Geometry check sheet. Reference: drawing and pictorial views, mm from the part's lowest x, y, z. A direction names the side the tool comes from. Give positions to 0.01 mm unless a question says otherwise; leave off trailing zeros. Loops run counter-clockwise (first coordinate to the right, second up) from the corner with the lowest first, then second, coordinate; pieces in that order, holes last. Notation, with made-up numbers: (30.5, 41.25) - (69.5, 41.25) arc R7 ccw to (69.5, 49.25) - close; hole circle Ø7 at (-36.75, -9). An arc over 180 degrees is marked (long way). Use CSV: the item, a comma, the result in double quotes.
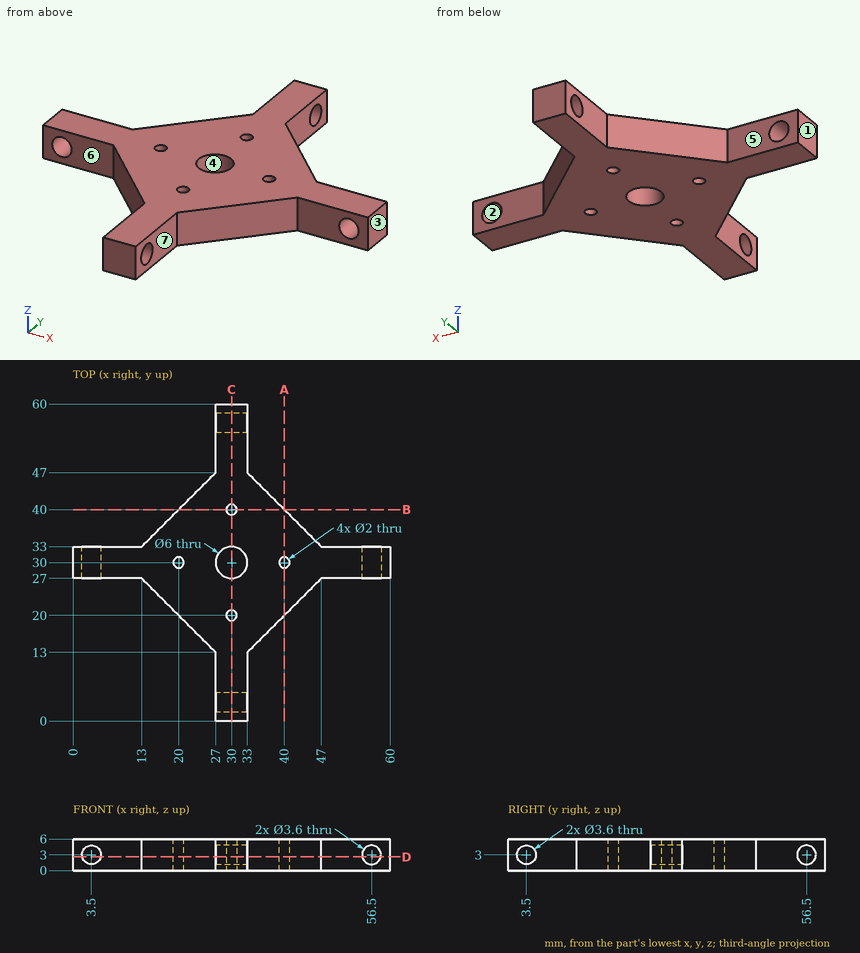
1. Set-up check for the marked faces 5, 6 and 7: record each of +Z, -Z, +X, -X, +Y, -Y from which the full face is reachable in a straight line by a thin tool's end or side.
Completed:
face 5,"+Z, -Z, -X, +Y"
face 6,"+Z, -Z, -X, -Y"
face 7,"+Z, -Z, +X, -Y"
2. Sectioned sample at C-C, the plane x = 30. Record the boundary of the cut face in (y, z).
Completed:
outline,"(0, 0) - (19, 0) - (19, 6) - (0, 6) - close; (21, 0) - (27, 0) - (27, 6) - (21, 6) - close; (33, 0) - (39, 0) - (39, 6) - (33, 6) - close; (41, 0) - (60, 0) - (60, 6) - (41, 6) - close; hole circle Ø3.6 at (3.5, 3); hole circle Ø3.6 at (56.5, 3)"
3. Sectioned sample at A-A, the plane x = 40. Record the boundary of the cut face in (y, z).
Completed:
outline,"(20, 0) - (29, 0) - (29, 6) - (20, 6) - close; (31, 0) - (40, 0) - (40, 6) - (31, 6) - close"
4. Scan lines: line 1 along Y through (x, z) = (30, 2.9); line 2 along X through (y, z) = (28.35, 3); line 3 along Y through (x, z) = (28.5, 3). Record each from-to range of solid material in increasing order.
Completed:
line 1,"y = 0 to 1.7, 5.3 to 19, 21 to 27, 33 to 39, 41 to 54.7, 58.3 to 60"
line 2,"x = 0 to 1.7, 5.3 to 27.49, 32.51 to 54.7, 58.3 to 60"
line 3,"y = 0 to 1.7, 5.3 to 27.4, 32.6 to 54.7, 58.3 to 60"
5. Sectioned sample at D-D, the plane z = 2.6. State how many separate pieces and enclosed holes the cut face has, and give its area (3 significant figures).
Completed:
separate pieces,"5"
enclosed holes,"5"
area,"951 mm²"
6. Go/stop test with flat-tipped pins: pin 1 Ø1.8 at (x, z) = (9, 2) entering from +Y; pin 2 Ø1.8 at (x, y) = (30, 40) entering from +Z; pin 3 Ø1.8 at (y, z) = (51, 2.5) entering from +X. Record where each tip stops, or that it passes through.
Completed:
pin 1,"stops at y = 33"
pin 2,"passes through"
pin 3,"stops at x = 33"
7. Release check for a two-part mould opening along X. For the marked faces 1, 2, 3 and 4 record: released by +X, released by -X, zero draft, split by the parting line, or undercut.
Completed:
face 1,"released by -X"
face 2,"undercut"
face 3,"released by +X"
face 4,"undercut"
